```python
from build123d import *

# Parameters (mm, degrees)
SALIENTE_EXTRUIR1_DEPTH      = 20
TALADRO_DE_MARGEN_PARA_M31_D = 3
CHAFL_N2_SIZE                = 1


with BuildPart() as part:
    # Croquis1 → Saliente-Extruir1 (new, symmetric)
    with BuildSketch(Plane(origin=(0, 0, 0), x_dir=(0, 1, 0), z_dir=(0, 0, 1))):
        Polygon((-6, 0), (6, 0), (6, 3), (4.5, 4.5), (4.5, 11.5), (2.5, 11.5), (2.5, 4.5), (-2.5, 4.5), (-2.5, 11.5), (-4.5, 11.5), (-4.5, 4.5), (-6, 3), align=None)
    extrude(amount=SALIENTE_EXTRUIR1_DEPTH, both=True)

    # Taladro de margen para M31 (through all)
    with Locations(Plane(origin=(0, 4.5, 0), x_dir=(-1, 0, 0), z_dir=(0, 1, 0))):
        with Locations((8, -10), (8, 10)):
            Hole(TALADRO_DE_MARGEN_PARA_M31_D / 2)

    # Chaflán2
    chafl_n2_edges = [part.edges().sort_by_distance(p)[0] for p in [
        (-11.5, -3.5, -20),
        (-11.5, 3.5, -20),
        (-11.5, 3.5, 20),
        (-11.5, -3.5, 20),
    ]]
    chamfer(chafl_n2_edges, length=CHAFL_N2_SIZE)


solid = part.part
```
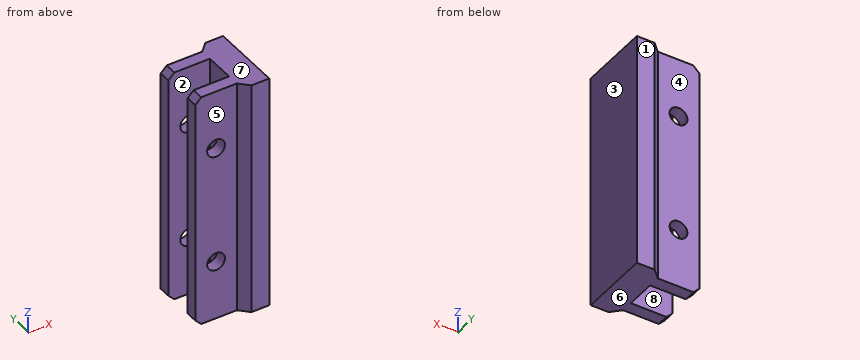
Check sheet for the modelled part. Datum: model origin and axes. Units: mm. Face numbers are marked on the shaded views. A direction names the side the tool comes from. Coordinates: 2 decimals unless noted, no trailing zeros. Write each loop counter-clockwise with the first axis right and the second up, starting at its lowest first coordinate (ties: lowest second). Pieces come first, ordered by that corner, then holes. Notation, with made-up numbers: (15, -15.5) - (56, -15.5) arc R28 cw to (56, 15.5) - close; hole circle Ø9 at (76, 63). An arc over 180 degrees is marked (long way). One line per question, with ' | ' between items.
Item 1: Thickness scan on line 1 (Z direction, x = -8, y = 3.65); line 2 (Y direction, x = -7, z = -7); line 3 (X direction, y = -2, z = -5). Record the ranges inside material, lowest first. Write a range as [from, to].
Determined:
line 1: z = [-20, -11.5], [-8.5, 8.5], [11.5, 20] | line 2: y = [-4.5, -2.5], [2.5, 4.5] | line 3: x = [-4.5, 0]
Item 2: Sectioned sample at D-D on y = -1.75. Record the boundary of the cut face in (x, z), plus the area to 3 significant figures.
Determined:
outline: (-4.5, -20) - (0, -20) - (0, 20) - (-4.5, 20) - close | area: 180 mm2
Item 3: Gauge pin test, flat ends, axial feed: P1, Ø2, axis at x = -6.5, z = -2, coming from the +Y side; P2, Ø4, axis at y = 1, z = 7, coming from the -X side; P3, Ø2, axis at x = -7.5, z = 2.5, coming from the -Y side; P4, Ø1, axis at x = -4, z = -11, coming from the +Y side. Record the tip position at first contact, or that the pin passes through.
Determined:
P1: stops at y = 4.5 | P2: stops at x = -11.5 | P3: stops at y = -4.5 | P4: stops at y = 5.5
Item 4: Sectioned sample at B-B on x = -8. Record the boundary of the cut face in (y, z), plus the area to 3 significant figures.
Determined:
outline: (-4.5, -20) - (-2.5, -20) - (-2.5, -11.5) - (-4.5, -11.5) - close; (-4.5, -8.5) - (-2.5, -8.5) - (-2.5, 8.5) - (-4.5, 8.5) - close; (-4.5, 11.5) - (-2.5, 11.5) - (-2.5, 20) - (-4.5, 20) - close; (2.5, -20) - (4.5, -20) - (4.5, -11.5) - (2.5, -11.5) - close; (2.5, -8.5) - (4.5, -8.5) - (4.5, 8.5) - (2.5, 8.5) - close; (2.5, 11.5) - (4.5, 11.5) - (4.5, 20) - (2.5, 20) - close | area: 136 mm2
Item 5: Mould release check, pull along Y, two halves, no side actions. Record for the marked faces 1, 2 and 3: pulls with the +Y half, pulls with the -Y half, needs draft (parallel to the pull), parting line crosses it, or undercut.
Determined:
face 1: pulls with the +Y half | face 2: undercut | face 3: needs draft
Item 6: Sectioned sample at A-A on z = 10. Record the boundary of the cut face in (x, y).
Determined:
outline: (-11.5, -4.5) - (-9.5, -4.5) - (-9.5, -2.5) - (-11.5, -2.5) - close; (-11.5, 2.5) - (-9.5, 2.5) - (-9.5, 4.5) - (-11.5, 4.5) - close; (-6.5, -4.5) - (-4.5, -4.5) - (-3, -6) - (0, -6) - (0, 6) - (-3, 6) - (-4.5, 4.5) - (-6.5, 4.5) - (-6.5, 2.5) - (-4.5, 2.5) - (-4.5, -2.5) - (-6.5, -2.5) - close
Item 7: Access from +Z, -Z, +X, -X, +Y, -Y to the whole of each face (thin tool, end or side, straight path). Record for the marked faces 4, 5, 6, 7 and 8.
Determined:
face 4: +Z, -Z, -X, +Y | face 5: +Z, -Z, -X, -Y | face 6: -Z, +X, -X, +Y, -Y | face 7: +Z, +X, -X, +Y, -Y | face 8: +Z, -Z, -X
Item 8: Sectioned sample at C-C on z = 1. Record the boundary of the cut face in (x, y).
Determined:
outline: (-11.5, -4.5) - (-4.5, -4.5) - (-3, -6) - (0, -6) - (0, 6) - (-3, 6) - (-4.5, 4.5) - (-11.5, 4.5) - (-11.5, 2.5) - (-4.5, 2.5) - (-4.5, -2.5) - (-11.5, -2.5) - close
